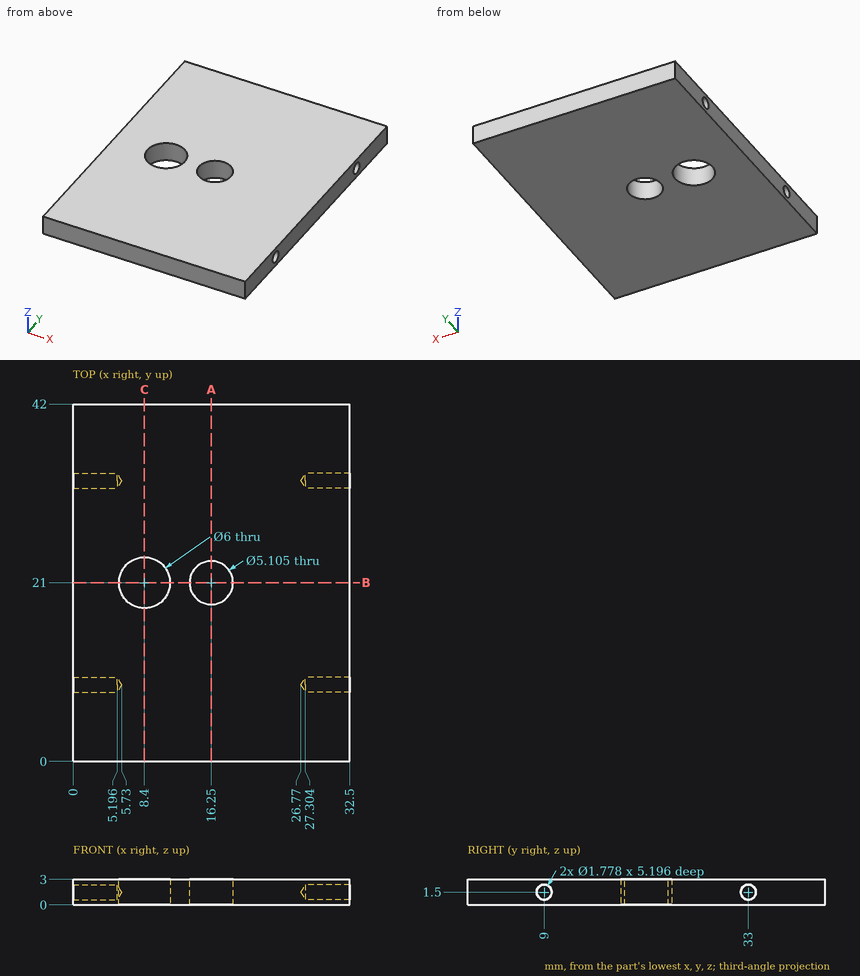
For this review, use the dimensioned drawing (mm, ordinates from the lowest corner) and the shaded views. Give positions to 0.01 mm unless a question says otherwise; leave off trailing zeros. Order: outer loops, then holes, each group sorted by start corner. A loop starts at its lowest first (then second) coordinate and runs counter-clockwise, first axis right, second up. Notation, with made-up numbers: (26, 63) - (36, 63) arc R9 ccw to (36, 75) - close; hole circle Ø4 at (66.5, 47). An arc over 180 degrees is marked (long way). Use a Markdown table: item, result. Add a question column.
(1) Add section B-B on y = 21. Give the boundary of the cut face in (x, z).
(2) Add section C-C on x = 8.4. Give the boundary of the cut face in (y, z).
(3) Clearance check with a flat-ended pin moving along its axis: P1, Ø1.4, axis at y = 9, z = 1.5, coming from the -X side. State where the tip first meets the part, or that it passes through.
(4) Add section A-A on x = 16.25. Give the boundary of the cut face in (y, z), then the cut area to 3 significant figures.
(5) Wall thickness on probe 1 along Y at (x, z) = (3.05, 1.5); probe 2 along Z at (x, y) = (28, 9); probe 3 along Y at (x, z) = (16.25, 1.9): over which ranges is each line inside the solid? List them lowest first. Write a range as [from, to].
Report:
| question | item | result |
|---|---|---|
| 1 | outline | (0, 0) - (5.4, 0) - (5.4, 3) - (0, 3) - close; (11.4, 0) - (13.7, 0) - (13.7, 3) - (11.4, 3) - close; (18.8, 0) - (32.5, 0) - (32.5, 3) - (18.8, 3) - close |
| 2 | outline | (0, 0) - (18, 0) - (18, 3) - (0, 3) - close; (24, 0) - (42, 0) - (42, 3) - (24, 3) - close |
| 3 | P1 | stops at x = 5.31 |
| 4 | outline | (0, 0) - (18.45, 0) - (18.45, 3) - (0, 3) - close; (23.55, 0) - (42, 0) - (42, 3) - (23.55, 3) - close |
| 4 | area | 111 mm² |
| 5 | probe 1 | y = [0, 8.11], [9.89, 32.11], [33.89, 42] |
| 5 | probe 2 | z = [0, 0.61], [2.39, 3] |
| 5 | probe 3 | y = [0, 18.45], [23.55, 42] |
